Read the model definition and answer for the solid it produces. Units are mm, in the model's axes. Face numbers are marked on the shaded views. A direction names the side the tool comes from. Coordinates: 2 decimals unless noted, no trailing zeros. Order: outer loops, then holes, each group sorted by start corner. A loop starts at its lowest first (then second) coordinate and runs counter-clockwise, first axis right, second up. Notation, with made-up numbers: (11.25, 43.25) - (22.25, 43.25) arc R19 cw to (22.25, 67.25) - close; hole circle Ø3 at (1, 79.5). An arc over 180 degrees is marked (long way). Use one line per item in the form item = value.
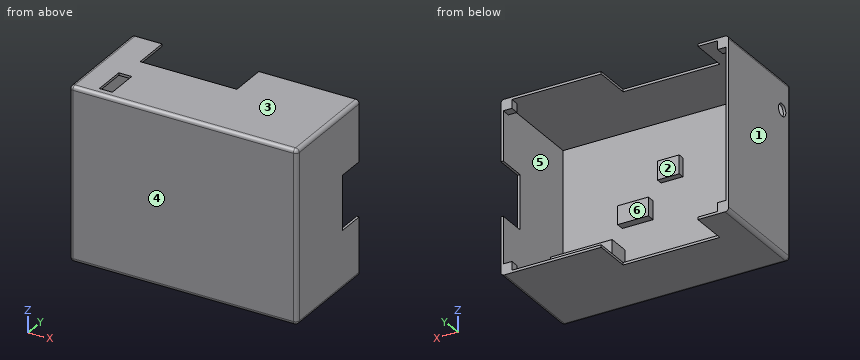
```python
from build123d import *

# Parameters (mm, degrees)
SKETCH1_W            = 185
SKETCH1_H            = 140
BOSS_EXTRUDE1_DEPTH  = 85
SKETCH2_W            = 181
SKETCH2_H            = 136
CUT_EXTRUDE1_DEPTH   = 82
CUT_EXTRUDE3_REACH   = 190.099
SKETCH3_W            = 60
SKETCH3_H            = 30
SKETCH6_W            = 7
SKETCH6_H            = 7
BOSS_EXTRUDE2_DEPTH  = 7
SKETCH7_W            = 7
SKETCH7_H            = 7
BOSS_EXTRUDE3_DEPTH  = 7
SKETCH8_W            = 7
SKETCH8_H            = 7
BOSS_EXTRUDE4_DEPTH  = 7
SKETCH9_W            = 7
SKETCH9_H            = 7
BOSS_EXTRUDE5_DEPTH  = 7
SKETCH11_W           = 50
SKETCH11_H           = 43
BOSS_EXTRUDE6_DEPTH  = 17.25
SKETCH12_W           = 25
SKETCH12_H           = 15
BOSS_EXTRUDE7_DEPTH  = 6.5
SKETCH13_W           = 10
SKETCH13_H           = 30
CUT_EXTRUDE4_DEPTH   = 174
SKETCH14_W           = 14
SKETCH14_H           = 25
BOSS_EXTRUDE8_DEPTH  = 5
SKETCH21_W           = 44
SKETCH21_H           = 23
CUT_EXTRUDE11_DEPTH  = 12
SKETCH23_R           = 5
CUT_EXTRUDE12_DEPTH  = 2
FILLET2_R            = 3
CUT_EXTRUDE13_START  = -140
SKETCH24_W           = 7
SKETCH24_H           = 30
CUT_EXTRUDE13_DEPTH  = 140
CUT_EXTRUDE14_START  = -140
SKETCH25_W           = 1.5
SKETCH25_H           = 30
CUT_EXTRUDE14_DEPTH  = 140
SKETCH26_W           = 17.682031304
SKETCH26_H           = 15.055987051
BOSS_EXTRUDE12_DEPTH = 5
SKETCH27_W           = 10.5
SKETCH27_H           = 26.5
CUT_EXTRUDE15_DEPTH  = 2


with BuildPart() as part:
    # Sketch1 → Boss-Extrude1 (new body)
    with BuildSketch(Plane(origin=(0, 0, 0), x_dir=(1, 0, 0), z_dir=(0, 1, 0))):
        Rectangle(SKETCH1_W, SKETCH1_H)
    extrude(amount=BOSS_EXTRUDE1_DEPTH)

    # Sketch2 → Cut-Extrude1 (cut)
    with BuildSketch(Plane(origin=(0, 85, 0), x_dir=(1, 0, 0), z_dir=(0, 1, 0))):
        Rectangle(SKETCH2_W, SKETCH2_H)
    extrude(amount=-CUT_EXTRUDE1_DEPTH, mode=Mode.SUBTRACT)

    # Cut-Extrude3: up to this face of the body (flat: up to its plane)
    cut_extrude3_end = Plane(part.part.faces().sort_by_distance((0, 42.5, -70))[0])
    # Sketch3 → Cut-Extrude3 (cut, up to the picked face)
    with BuildSketch(Plane.XY.offset(70), mode=Mode.PRIVATE) as cut_extrude3_sk1:
        with Locations((-37.5, 70)):
            Rectangle(SKETCH3_W, SKETCH3_H)
    cut_extrude3_tool1 = split(extrude(cut_extrude3_sk1.sketch, amount=-CUT_EXTRUDE3_REACH, mode=Mode.PRIVATE), bisect_by=cut_extrude3_end, keep=Keep.BOTH, mode=Mode.PRIVATE)
    add(cut_extrude3_tool1.solids().sort_by(Axis((-37.5, 70, 70), (0, 0, -1)))[0], mode=Mode.SUBTRACT)

    # Sketch6 → Boss-Extrude2 (add)
    with BuildSketch(Plane(origin=(0, 0, 68), x_dir=(-1, 0, 0), z_dir=(0, 0, -1))):
        with Locations((87, 81.5)):
            Rectangle(SKETCH6_W, SKETCH6_H)
    extrude(amount=BOSS_EXTRUDE2_DEPTH)

    # Sketch7 → Boss-Extrude3 (add)
    with BuildSketch(Plane.XY.offset(-68)):
        with Locations((-87, 81.5)):
            Rectangle(SKETCH7_W, SKETCH7_H)
    extrude(amount=BOSS_EXTRUDE3_DEPTH)

    # Sketch8 → Boss-Extrude4 (add)
    with BuildSketch(Plane(origin=(0, 0, 68), x_dir=(-1, 0, 0), z_dir=(0, 0, -1))):
        with Locations((-87, 81.5)):
            Rectangle(SKETCH8_W, SKETCH8_H)
    extrude(amount=BOSS_EXTRUDE4_DEPTH)

    # Sketch9 → Boss-Extrude5 (add)
    with BuildSketch(Plane.XY.offset(-68)):
        with Locations((87, 81.5)):
            Rectangle(SKETCH9_W, SKETCH9_H)
    extrude(amount=BOSS_EXTRUDE5_DEPTH)

    # Sketch11 → Boss-Extrude6 (add)
    with BuildSketch(Plane(origin=(0, 3, 0), x_dir=(1, 0, 0), z_dir=(0, 1, 0))):
        with Locations((65.5, 46.5)):
            Rectangle(SKETCH11_W, SKETCH11_H)
    extrude(amount=BOSS_EXTRUDE6_DEPTH)

    # Sketch12 → Boss-Extrude7 (add)
    with BuildSketch(Plane(origin=(0, 3, 0), x_dir=(1, 0, 0), z_dir=(0, 1, 0))):
        with Locations((30, 0)):
            Rectangle(SKETCH12_W, SKETCH12_H)
    extrude(amount=BOSS_EXTRUDE7_DEPTH)

    # Sketch13 → Cut-Extrude4 (cut)
    with BuildSketch(Plane.XY.offset(70)):
        with Locations((-2.5, 70)):
            Rectangle(SKETCH13_W, SKETCH13_H)
    extrude(amount=-CUT_EXTRUDE4_DEPTH, mode=Mode.SUBTRACT)

    # Sketch14 → Boss-Extrude8 (add)
    with BuildSketch(Plane(origin=(-90.5, 0, 0), x_dir=(0, 0, -1), z_dir=(1, 0, 0))):
        with Locations((0, 15.5)):
            Rectangle(SKETCH14_W, SKETCH14_H)
    extrude(amount=BOSS_EXTRUDE8_DEPTH)

    # Sketch21 → Cut-Extrude11 (cut)
    with BuildSketch(Plane(origin=(92.5, 0, 0), x_dir=(0, 0, -1), z_dir=(1, 0, 0))):
        with Locations((1, 73.5)):
            Rectangle(SKETCH21_W, SKETCH21_H)
    extrude(amount=-CUT_EXTRUDE11_DEPTH, mode=Mode.SUBTRACT)

    # Sketch23 → Cut-Extrude12 (cut)
    with BuildSketch(Plane.ZY.offset(92.5)):
        with Locations((44.895607786, 11.841525816)):
            Circle(SKETCH23_R)
    extrude(amount=-CUT_EXTRUDE12_DEPTH, mode=Mode.SUBTRACT)

    # Fillet2
    fillet2_edges = [part.edges().sort_by_distance(p)[0] for p in [
        (0, 0, -70),
        (92.5, 0, 0),
        (0, 0, 70),
        (-92.5, 0, 0),
        (-92.5, 42.5, -70),
        (92.5, 42.5, -70),
        (92.5, 42.5, 70),
        (-92.5, 42.5, 70),
    ]]
    fillet(fillet2_edges, radius=FILLET2_R)

    # Sketch24 → Cut-Extrude13 (cut)
    with BuildSketch(Plane(origin=(0, 0, -70), x_dir=(-1, 0, 0), z_dir=(0, 0, -1)).offset(CUT_EXTRUDE13_START)):
        with Locations((-6, 70)):
            Rectangle(SKETCH24_W, SKETCH24_H)
    extrude(amount=CUT_EXTRUDE13_DEPTH, mode=Mode.SUBTRACT)

    # Sketch25 → Cut-Extrude14 (cut)
    with BuildSketch(Plane(origin=(0, 0, -70), x_dir=(-1, 0, 0), z_dir=(0, 0, -1)).offset(CUT_EXTRUDE14_START)):
        with Locations((-10.25, 70)):
            Rectangle(SKETCH25_W, SKETCH25_H)
    extrude(amount=CUT_EXTRUDE14_DEPTH, mode=Mode.SUBTRACT)

    # Sketch26 → Boss-Extrude12 (add)
    with BuildSketch(Plane(origin=(0, 3, 0), x_dir=(1, 0, 0), z_dir=(0, 1, 0))):
        with Locations((2.188370211, -27.472006474)):
            Rectangle(SKETCH26_W, SKETCH26_H)
    extrude(amount=BOSS_EXTRUDE12_DEPTH)

    # Sketch27 → Cut-Extrude15 (cut)
    with BuildSketch(Plane.XY.offset(70)):
        with Locations((-66.878682152, 20.25)):
            Rectangle(SKETCH27_W, SKETCH27_H)
    extrude(amount=-CUT_EXTRUDE15_DEPTH, mode=Mode.SUBTRACT)


solid = part.part
```
(1) Straight lines are drawn through the part: L1, parallel to Z at x = -77, y = 53.5; L2, parallel to X at y = 47.5, z = 47.5; L3, parallel to X at y = 20, z = -63. For each, find the intervals that lie inside material, in ascending order.
Answer list:
L1 = -70 to -68, 68 to 70
L2 = -92.5 to -90.5, 90.5 to 92.5
L3 = -92.5 to -90.5, 40.5 to 92.5
(2) Section D-D, the plane y = 58.5 is taken. Write down the section's boundary in (x, z), then the cut area to 3 significant figures.
Answer list:
outline = (-92.5, -67) arc R3 ccw to (-89.5, -70) - (-67.5, -70) - (-67.5, -68) - (-90.5, -68) - (-90.5, 68) - (-67.5, 68) - (-67.5, 70) - (-89.5, 70) arc R3 ccw to (-92.5, 67) - close; (11, -70) - (89.5, -70) arc R3 ccw to (92.5, -67) - (92.5, 67) arc R3 ccw to (89.5, 70) - (11, 70) - (11, 68) - (90.5, 68) - (90.5, -68) - (11, -68) - close
area = 962 mm2
(3) Section A-A, the plane y = 68.5 is taken. Write down the section's boundary in (x, z).
Answer list:
outline = (-92.5, -67) arc R3 ccw to (-89.5, -70) - (-67.5, -70) - (-67.5, -68) - (-90.5, -68) - (-90.5, 68) - (-67.5, 68) - (-67.5, 70) - (-89.5, 70) arc R3 ccw to (-92.5, 67) - close; (11, -70) - (89.5, -70) arc R3 ccw to (92.5, -67) - (92.5, -23) - (90.5, -23) - (90.5, -68) - (11, -68) - close; (11, 68) - (90.5, 68) - (90.5, 21) - (92.5, 21) - (92.5, 67) arc R3 ccw to (89.5, 70) - (11, 70) - close
(4) Which of the six approach directions +Z, -Z, +X, -X, +Y, -Y give full straight-line access (tool end or side, diameter ignored) to the marked faces 4, 5 and 6?
Answer list:
face_4 = +Z, -Z, +X, -X, -Y
face_5 = none
face_6 = +Y
(5) Section C-C, the plane z = -18.5 is taken. Write down the section's boundary in (x, y), then the cut area to 3 significant figures.
Answer list:
outline = (-92.5, 3) arc R3 ccw to (-89.5, 0) - (89.5, 0) arc R3 ccw to (92.5, 3) - (92.5, 62) - (90.5, 62) - (90.5, 3) - (-90.5, 3) - (-90.5, 85) - (-92.5, 85) - close
area = 833 mm2
(6) Given pin 1 Ø1 at (y, z) = (18.5, 69.5) entering from -X; pin 2 Ø2 at (y, z) = (15.5, 69) entering from +X; pin 3 Ø7.5 at (x, z) = (32.5, 0) entering from +Y, each flat-ended and moving along its own axis, determine where each tip first touches the part or whether it passes through.
Answer list:
pin_1 = -91.74
pin_2 = 92.33
pin_3 = 9.5
(7) The mould has two halves that part along Z. Classify the marked faces 1, 2 and 3: +Z half, -Z half, draft (parallel to the pull), parting line (faces both ways), or undercut.
Answer list:
face_1 = draft
face_2 = undercut
face_3 = +Z half
(8) Section B-B, the plane y = 35.5 is taken. Write down the section's boundary in (x, z).
Answer list:
outline = (-92.5, -67) arc R3 ccw to (-89.5, -70) - (89.5, -70) arc R3 ccw to (92.5, -67) - (92.5, 67) arc R3 ccw to (89.5, 70) - (-89.5, 70) arc R3 ccw to (-92.5, 67) - close; hole (-90.5, -68) - (90.5, -68) - (90.5, 68) - (-90.5, 68) - close
